Source: CAD feature listing. Evaluate the final solid. Frame: model axes, mm. A direction names the side the tool comes from. Give positions to 0.01 mm unless a question says otherwise; leave off trailing zeros. Write each loop counter-clockwise with the first axis right and the second up, starting at its lowest first coordinate (ties: lowest second). Pieces come first, ordered by that corner, then holes. Notation, with made-up numbers: M 42.5,-32 L 70.5,-32 A8 ccw 70.5,-25 Z; hole C 51,-39.75 d9. An arc over 180 degrees is marked long. Answer as a JSON object with one key per item and string values. Group by question number.
Autodesk Fusion 360 part; units mm, degrees
sketch "Szkic1" plane through (0, 0, 0) normal (0, 0, 1) x (1, 0, 0)
  line L0 (29, -110) -> (29, -70)
  line L1 (-10, -75) -> (10, -75)
  line L2 (10, -75) -> (10, -98.8)
  line L3 (-45, -110) -> (29, -110)
  circle A0 centre (15, -80) radius 3.5
  circle A1 centre (15, -100) radius 3.5
  line L4 (-10, -98.8) -> (-10, -75)
  line L5 (10, -98.8) -> (-10, -98.8)
  circle A2 centre (-20, -100) radius 3.5
  circle A3 centre (-20, -80) radius 3.5
  line L6 (29, -70) -> (35, -70)
  line L7 (35, -70) -> (35, 160)
  circle A4 centre (25, -50) radius 1.75
  circle A5 centre (25, 0) radius 1.75
  circle A6 centre (25, 50) radius 1.75
  circle A7 centre (25, 100) radius 1.75
  line L8 (35, 160) -> (-45, 160)
  circle A8 centre (25, 150) radius 1.75
  circle A9 centre (-25, 150) radius 1.75
  line L9 (35, 160) -> (35, 135)
  line L10 (35, 135) -> (-45, 135)
  line L11 (-45, 135) -> (-45, 160)
  line L12 (-45, 160) -> (35, 160)
  line L13 (35, 135) -> (35, -70)
  line L14 (35, -70) -> (17, -70)
  line L15 (17, -70) -> (17, 135)
  line L16 (17, 135) -> (35, 135)
  line L17 (17, 135) -> (17, -70)
  line L18 (17, -70) -> (12, -70)
  line L19 (12, -70) -> (12, 135)
  line L20 (12, 135) -> (17, 135)
  dimension "d1" = 25
  dimension "d2" = 18
  dimension "d3" = 5
extrude "Wyciągnięcie proste1" add sketch "Szkic1" along normal blind 15 contours L6 L7 L10 L13 L14 L15 L16 L17
extrude "Wyciągnięcie proste2" add sketch "Szkic1" along normal blind 25 contours L10 L15 L17 L18 L19 L20
extrude "Wyciągnięcie proste3" add 1 faces at (21.3333, 135, 5) along direction (0, 1, 0) blind 26
extrude "Wyciągnięcie proste4" cut sketch "Szkic1" along normal blind 27 contours A8
sketch "Szkic2" plane through (0, 0, 0) normal (0, 0, -1) x (1, 0, 0)
  circle A0 centre (25, -150) radius 1.75
  circle A1 centre (25, -50) radius 1.75
  circle A2 centre (25, -100) radius 1.75
  circle A3 centre (25, 0) radius 1.75
  circle A4 centre (25, 50) radius 1.75
  line L0 (35, -161) -> (35, 70)
  line L1 (35, 70) -> (12, 70)
  line L2 (12, 70) -> (12, -161)
  line L3 (12, -161) -> (35, -161)
  circle A5 centre (25, -150) radius 3.5
  circle A6 centre (25, -100) radius 2
  circle A7 centre (25, -50) radius 2
  circle A8 centre (25, 0) radius 2
  circle A9 centre (25, 50) radius 2
  dimension "d12" = 7
  dimension "d13" = 4
  dimension "d14" = 4
  dimension "d15" = 4
  dimension "d16" = 4
extrude "Wyciągnięcie proste5" cut sketch "Szkic2" against normal blind 100 contours A6 | A7 | A8 | A9
extrude "Wyciągnięcie proste6" cut sketch "Szkic2" against normal blind 4 contours A5
sketch "Szkic3" plane through (0, 0, 0) normal (0, 0, -1) x (1, 0, 0)
  circle A0 centre (25, -150) radius 2
  dimension "d21" = 4
extrude "Wyciągnięcie proste7" cut sketch "Szkic3" against normal blind 100
(1) Section D-D, the plane z = 20.25. Return loops of the section in (x, y).
(2) Contact query for flat-ended pins moving along their axis: pin 1 Ø5.5 at (x, y) = (28.5, 49) entering from +Z; pin 2 Ø2 at (x, y) = (26, 149.5) entering from -Z. Output: stop coordinate, or through.
(3) Access query for faces 4 (the flat face through (27, 152, 4)), 5 (the cylindrical face through (25, 52, 7)), 6 (the flat face through (26, 44, 15)). Directions: +Z, -Z, +X, -X, +Y, -Y. A direction counts if a zero-diameter tool reaches every point of the face in a straight line with its end or side. Return the directions, or none.
(4) Pull-direction query (Y, two-part tool) for faces 1 (the flat face through (21, -70, 10)), 2 (the cylindrical face through (25.923, 151.774, 9.423)), 3 (the flat face through (15, 44, 25)); classes: pulls with the +Y half, pulls with the -Y half, needs draft (parallel to the pull), parting line crosses it, or undercut.
(5) Ray query, L1, parallel to Y at x = 25, z = 8; L2, parallel to Y at x = 25, z = 3.75; L3, parallel to X at y = 0, z = 10.75. Return the intervals inside material, ascending. Write a range as [from, to].
(6) Section A-A, the plane y = -50. Return loops of the section in (x, z), plus the area to 3 significant figures.
(7) Section B-B, the plane x = 25. Return loops of the section in (y, z), plus the area to 3 significant figures.
(8) Section C-C, the plane y = 69.5. Return loops of the section in (x, z), plus the area to 3 significant figures.
Reported:
{
 "1": {"outline": "M 12,-70 L 17,-70 L 17,161 L 12,161 Z"},
 "2": {"pin 1": "stops at z = 15", "pin 2": "stops at z = 4"},
 "3": {"face 4": "-Z", "face 5": "+Z, -Z", "face 6": "+Z, +X, +Y, -Y"},
 "4": {"face 1": "pulls with the -Y half", "face 2": "undercut", "face 3": "needs draft"},
 "5": {"L1": "y = [-70, -52], [-48, -2], [2, 48], [52, 98], [102, 148], [152, 161]", "L2": "y = [-70, -52], [-48, -2], [2, 48], [52, 98], [102, 146.5], [153.5, 161]", "L3": "x = [12, 23], [27, 35]"},
 "6": {"outline": "M 12,0 L 23,0 L 23,15 L 17,15 L 17,25 L 12,25 Z; M 27,0 L 35,0 L 35,15 L 27,15 Z", "area": "335 mm2"},
 "7": {"outline": "M -70,0 L -52,0 L -52,15 L -70,15 Z; M -48,0 L -2,0 L -2,15 L -48,15 Z; M 2,0 L 48,0 L 48,15 L 2,15 Z; M 52,0 L 98,0 L 98,15 L 52,15 Z; M 102,0 L 146.5,0 L 146.5,4 L 148,4 L 148,15 L 102,15 Z; M 152,4 L 153.5,4 L 153.5,0 L 161,0 L 161,15 L 152,15 Z", "area": "3,150 mm2"},
 "8": {"outline": "M 12,0 L 35,0 L 35,15 L 17,15 L 17,25 L 12,25 Z", "area": "395 mm2"}
}
